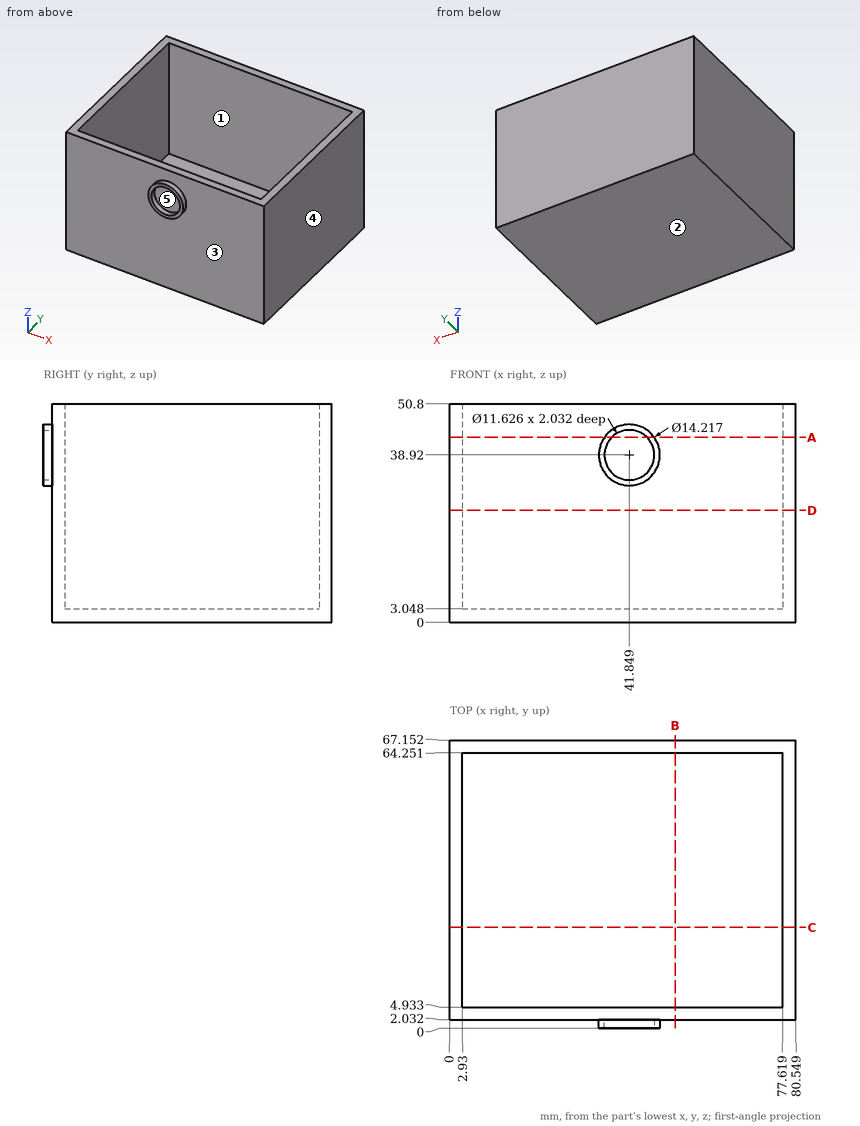
Check sheet for the drawn part. Datum: minimum x, y, z corner. Units: mm. A direction names the side the tool comes from. Round coordinates to 2 decimals unless told otherwise and drop trailing zeros. Loops run counter-clockwise (first coordinate to the right, second up) from the corner with the lowest first, then second, coordinate; pieces in that order, holes last. Notation, with made-up numbers: M 33,64.25 L 57,64.25 A33 cw 57,95.25 Z; hole C 44,35 d1. An arc over 180 degrees is marked long. One line per question, with ' | ' between items. Start each with the question number.
Item 1: Section check B-B (x = 52.5). Record the boundary of the cut face in (y, z).
Item 2: Set-up check for the marked faces 1 and 2: record each of +Z, -Z, +X, -X, +Y, -Y from which the full face is reachable in a straight line by a thin tool's end or side.
Item 3: Section check D-D (z = 26). Record the boundary of the cut face in (x, y), and give its area (3 significant figures).
Item 4: Scan lines: probe 1 along Y at (x, z) = (27, 26); probe 2 along X at (y, z) = (58, 37); probe 3 along Z at (x, y) = (55.5, 13.5). Record each from-to range of solid material in increasing order.
Item 5: Section check C-C (y = 23.5). Record the boundary of the cut face in (x, z).
Item 6: Release check for a two-part mould opening along X. For the marked faces 3, 4 and 5 record: released by +X, released by -X, zero draft, split by the parting line, or undercut.
Item 7: Gauge pin test, flat end, axial feed: pin 1 Ø6 at (x, y) = (27.5, 28) entering from +Z. Record the tip position at first contact, or that the pin passes through.
Item 8: Section check A-A (z = 43). Record the boundary of the cut face in (x, y).
Worked out:
1) outline: M 2.03,0 L 67.15,0 L 67.15,50.8 L 64.25,50.8 L 64.25,3.05 L 4.93,3.05 L 4.93,50.8 L 2.03,50.8 Z
2) face 1: +Z | face 2: -Z, +X, -X, +Y, -Y
3) outline: M 0,2.03 L 80.55,2.03 L 80.55,67.15 L 0,67.15 Z; hole M 2.93,4.93 L 77.62,4.93 L 77.62,64.25 L 2.93,64.25 Z | area: 815 mm^2
4) probe 1: 2.03 to 4.93, 64.25 to 67.15 | probe 2: 0 to 2.93, 77.62 to 80.55 | probe 3: 0 to 3.05
5) outline: M 0,0 L 80.55,0 L 80.55,50.8 L 77.62,50.8 L 77.62,3.05 L 2.93,3.05 L 2.93,50.8 L 0,50.8 Z
6) face 3: zero draft | face 4: released by +X | face 5: undercut
7) pin 1: z = 3.05
8) outline: M 0,2.03 L 36.03,2.03 L 36.03,0 L 37.71,0 L 37.71,2.03 L 45.99,2.03 L 45.99,0 L 47.67,0 L 47.67,2.03 L 80.55,2.03 L 80.55,67.15 L 0,67.15 Z; hole M 2.93,4.93 L 77.62,4.93 L 77.62,64.25 L 2.93,64.25 Z
